```python
from build123d import *

# Parameters (mm, degrees)
F0_R     = 11.25
F0_R_2   = 6.197174
F0_R_3   = 11.255413
F0_R_4   = 11
F1_DEPTH = 9


with BuildPart() as f1:
    # F0 (on Top) → F1 (new body)
    with BuildSketch(Plane.XY):
        with BuildLine():
            Line((-18.857145, -28.667178), (18.857145, -28.667178))
            ThreePointArc((18.857145, -28.667178), (34.255077, -19.777178), (34.255077, -1.997178))
            Line((34.255077, -1.997178), (15.397932, 30.664356))
            ThreePointArc((15.397932, 30.664356), (0, 39.554356), (-15.397932, 30.664356))
            Line((-15.397932, 30.664356), (-34.255077, -1.997178))
            ThreePointArc((-34.255077, -1.997178), (-34.255077, -19.777178), (-18.857145, -28.667178))
        make_face()
        with Locations((-21.997045, -12.7)):
            Circle(F0_R, mode=Mode.SUBTRACT)
        with Locations((0, -19.717751)):
            Circle(F0_R_2, mode=Mode.SUBTRACT)
        Circle(F0_R, mode=Mode.SUBTRACT)
        with Locations((21.997045, -12.7)):
            Circle(F0_R_3, mode=Mode.SUBTRACT)
        with Locations((-17.076073, 9.858875)):
            Circle(F0_R_2, mode=Mode.SUBTRACT)
        with Locations((0, 25.4)):
            Circle(F0_R_4, mode=Mode.SUBTRACT)
        with Locations((17.076073, 9.858875)):
            Circle(F0_R_2, mode=Mode.SUBTRACT)
    extrude(amount=F1_DEPTH)


solid = f1.part
```
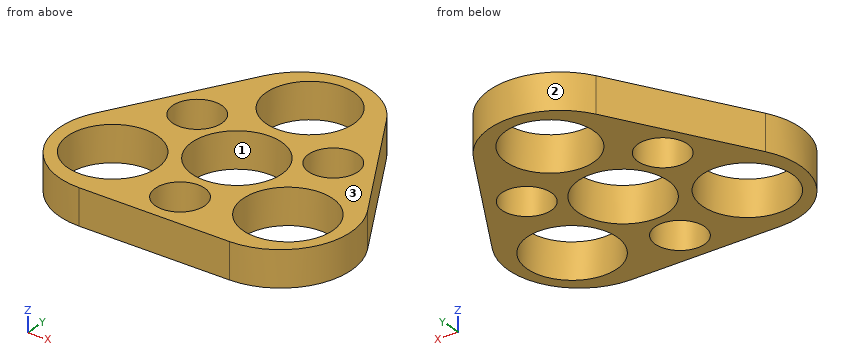
Model file for the job. Use its own axes, mm. Face numbers are marked on the shaded views. Give positions to 0.01 mm unless a question says otherwise; leave off trailing zeros. Loops run counter-clockwise (first coordinate to the right, second up) from the corner with the lowest first, then second, coordinate; pieces in that order, holes last. Notation, with made-up numbers: (53, 10) - (110, 10) arc R19 cw to (110, 29) - close; hole circle Ø4 at (34.5, -9). An arc over 180 degrees is marked (long way). One line per item, written item: value. Start each with the question number.
1. Slice it at B-B (y = -12.7). List the corners of the cut face in (x, z), plus the area to 3 significant figures.
2. Pull direction X, two halves, no side cores. Call the marked faces 1, 2 and 3: pulls with the +X half, pulls with the -X half, needs draft (parallel to the pull), parting line crosses it, or undercut.
3. Pin check, flat tips, straight feed: pin 1 (5 mm diameter, centred on y = 24, z = 2, fed in from +X); pin 2 (5 mm diameter, centred on x = 26.5, z = 7, fed in from +Y); pin 3 (1 mm diameter, centred on y = 27, z = 3.5, fed in from +X). Stop position of each tip, or through.
4. Slice it at C-C (z = 3.25). List the corners of the cut face in (x, y).
5. Slice it at A-A (x = 0). List the corners of the cut face in (y, z).
6. Probe L1, parallel to Y at x = 0, z = 3.75; L2, parallel to Y at x = 12.5, z = 4; L3, parallel to X at y = -20.5, z = 2.75. List the from-to ranges inside material, lowest first. Write a range as from..to.
7. Slice it at D-D (x = -29.5). List the corners of the cut face in (y, z).
Solution:
1. outline: (-36.54, 0) - (-33.25, 0) - (-33.25, 9) - (-36.54, 9) - close; (-10.75, 0) - (10.74, 0) - (10.74, 9) - (-10.75, 9) - close; (33.25, 0) - (36.54, 0) - (36.54, 9) - (33.25, 9) - close
1. area: 253 mm^2
2. face 1: undercut
2. face 2: parting line crosses it
2. face 3: needs draft
3. pin 1: stops at x = 20.69
3. pin 2: stops at y = 15.77
3. pin 3: stops at x = 17.8
4. outline: (-34.26, -2) arc R17.78 ccw to (-18.86, -28.67) - (18.86, -28.67) arc R17.78 ccw to (34.26, -2) - (15.4, 30.66) arc R17.78 ccw to (-15.4, 30.66) - close; hole circle Ø22.5 at (-22, -12.7); hole circle Ø12.39 at (-17.08, 9.86); hole circle Ø22.5 at (0, 0); hole circle Ø22 at (0, 25.4); hole circle Ø12.39 at (0, -19.72); hole circle Ø22.51 at (22, -12.7); hole circle Ø12.39 at (17.08, 9.86)
5. outline: (-28.67, 0) - (-25.91, 0) - (-25.91, 9) - (-28.67, 9) - close; (-13.52, 0) - (-11.25, 0) - (-11.25, 9) - (-13.52, 9) - close; (11.25, 0) - (14.4, 0) - (14.4, 9) - (11.25, 9) - close; (36.4, 0) - (39.55, 0) - (39.55, 9) - (36.4, 9) - close
6. L1: y = -28.67..-25.91, -13.52..-11.25, 11.25..14.4, 36.4..39.55
6. L2: y = -28.67..-18.74, -6.66..5.68, 14.04..34.42
6. L3: x = -33.81..-30.1, -13.89..-6.15, 6.15..13.88, 30.11..33.81
7. outline: (-25.13, 0) - (-21.08, 0) - (-21.08, 9) - (-25.13, 9) - close; (-4.32, 0) - (6.24, 0) - (6.24, 9) - (-4.32, 9) - close
